Geometry check sheet. Reference: the model listing, model coordinates, mm. Round coordinates to 2 decimals unless told otherwise and drop trailing zeros. Write each loop counter-clockwise with the first axis right and the second up, starting at its lowest first coordinate (ties: lowest second). Pieces come first, ordered by that corner, then holes.
Item 1: Depth check by flat-ended pin: P1, Ø0.9, axis at y = -156, z = 1.5, coming from the +X side. Enter the tip coordinate at first touch or a pass-through.
Item 2: Scan lines: probe 1 along Y at (x, z) = (32.5, 2); probe 2 along Y at (x, z) = (8, 1.5); probe 3 along X at (y, z) = (-145, 2.05). Record each from-to range of solid material in increasing order.
Item 3: Cross-section at A-A (x = 46). Enter the section's corners in (y, z).
Item 4: Cross-section at B-B (y = -121.5). Enter the section's corners in (x, z).
Item 5: Cross-section at C-C (z = 1). State how many separate pieces and enclosed holes the cut face has, then the cut area to 3 significant figures.
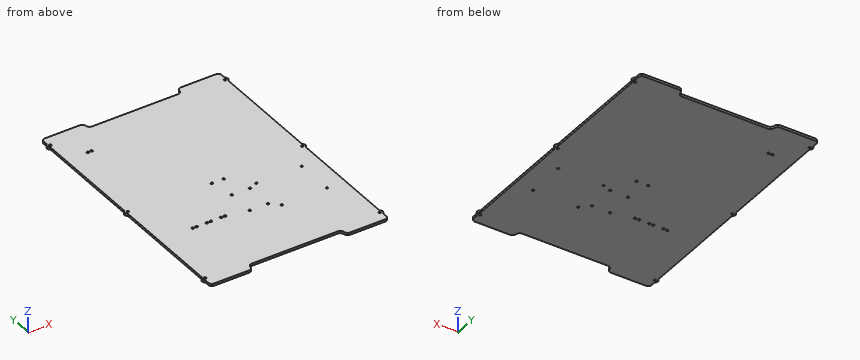
Autodesk Inventor part; units mm, degrees
ref_plane "YZ Plane" through (0, 0, 0) normal (1, 0, 0) x (0, 1, 0)
ref_plane "XZ Plane" through (0, 0, 0) normal (0, 1, 0) x (-1, 0, 0)
ref_plane "XY Plane" through (0, 0, 0) normal (0, 0, 1) x (1, 0, 0)
sketch "Sketch1" plane through (0, 0, 0) normal (0, 0, 1) x (1, 0, 0)
  line L0 (-114, -164) -> (114, -164)
  line L1 (114, 164) -> (-114, 164)
  line L2 (-114, -164) -> (114, 164) construction
  line L3 (114, -164) -> (-114, 164) construction
  line L4 (-112, -150) -> (112, -150)
  line L5 (112, -150) -> (112, 150)
  line L6 (112, 150) -> (-112, 150)
  line L7 (-112, 150) -> (-112, -150)
  line L8 (-112, -150) -> (112, 150) construction
  line L9 (112, -150) -> (-112, 150) construction
  circle A0 centre (112, 150) radius 1.5
  arc A1 (114, 146.5359) -> (114, 153.4641) centre (112, 150) ccw
  line L10 (114, 153.4641) -> (114, 164)
  line L11 (0, -56.7016) -> (0, 56.7016)
  line L12 (-37.0034, 0) -> (37.0034, 0)
  circle A2 centre (-112, 150) radius 1.5
  arc A3 (-114, 153.4641) -> (-114, 146.5359) centre (-112, 150) ccw
  circle A4 centre (112, -150) radius 1.5
  arc A5 (114, -153.4641) -> (114, -146.5359) centre (112, -150) ccw
  arc A6 (-114, -146.5359) -> (-114, -153.4641) centre (-112, -150) ccw
  circle A7 centre (-112, -150) radius 1.5
  line L13 (-114, 164) -> (-114, 153.4641)
  line L14 (114, -164) -> (114, -153.4641)
  line L15 (-114, -153.4641) -> (-114, -164)
  circle A8 centre (112, 0) radius 1.5
  arc A9 (114, -3.4641) -> (114, 3.4641) centre (112, 0) ccw
  line L16 (114, -146.5359) -> (114, -3.4641)
  line L17 (114, 3.4641) -> (114, 146.5359)
  circle A10 centre (-112, 0) radius 1.5
  arc A11 (-114, 3.4641) -> (-114, -3.4641) centre (-112, 0) ccw
  line L18 (-114, 146.5359) -> (-114, 3.4641)
  line L19 (-114, -3.4641) -> (-114, -146.5359)
  line L20 (-60, 164) -> (60, 164)
  line L21 (60, 164) -> (-60, 164)
  line L22 (-60, 164) -> (-60, 155)
  line L23 (-60, 155) -> (60, 155)
  line L24 (60, 155) -> (60, 164)
  line L25 (-60, -164) -> (-60, -155)
  line L26 (-60, -155) -> (60, -155)
  line L27 (60, -155) -> (60, -164)
  point P0 (0, 0)
  point P1 (0, 164)
  dimension "d0" = 228
  dimension "d1" = 328
  dimension "d2" = 224
  dimension "d3" = 300
  dimension "d4" = 3
  dimension "d10" = 3
  dimension "d11" = 8
  dimension "d12" = 120
  dimension "d13" = 120
  dimension "d14" = 9
extrude "Extrusion1" add sketch "Sketch1" along normal blind 3 contours L15 A6 L19 A11 L18 A3 L13 L1 L22 L23 L24 L10 A1 L17 A9 L16 A5 L14 L0 L27 L26 L25 | A7 L7 A10 A2 L6 A0 L5 A8 A4 L4
fillet "Fillet1" radius 4.1 4 edges at (114, 164, 1.5) (114, -164, 1.5) (-114, 164, 1.5) (-114, -164, 1.5)
fillet "Fillet2" radius 5 8 edges at (-60, 164, 1.5) (60, 164, 1.5) (60, 155, 1.5) (-60, 155, 1.5) (-60, -164, 1.5) (-60, -155, 1.5) (60, -155, 1.5) (60, -164, 1.5)
sketch "Sketch3" plane through (0, 0, 3) normal (0, 0, 1) x (1, 0, 0)
  circle A0 centre (-66.131, -64.28) radius 1.5
  circle A1 centre (-71.131, -64.28) radius 1.5
  circle A2 centre (-52.931, -64.28) radius 1.5
  circle A3 centre (-47.931, -64.28) radius 1.5
  circle A4 centre (-34.731, -64.28) radius 1.5
  circle A5 centre (-29.731, -64.28) radius 1.5
  circle A6 centre (-1.75, -35.23) radius 1.45
  circle A7 centre (21.55, -35.23) radius 1.45
  circle A8 centre (-1.75, -70.23) radius 1.45
  circle A9 centre (21.55, -70.23) radius 1.45
  circle A10 centre (32.5, -80.28) radius 1.35
  circle A11 centre (32.5, -31.28) radius 1.35
  circle A12 centre (90.5, -80.28) radius 1.35
  circle A13 centre (90.5, -31.28) radius 1.35
  circle A14 centre (-86.131, 116.72) radius 1.5
  circle A15 centre (-81.131, 116.72) radius 1.5
  circle A16 centre (-7.4766, -5.121) radius 1.5084
  circle A17 centre (7.5843, -5.1439) radius 1.4324
  point P0 (0, 0)
extrude "Extrusion3" cut sketch "Sketch3" against normal blind 3
properties part number "Control layer"
Resolved:
1. P1: stops at x = 114
2. probe 1: y = -155 to -81.63, -78.93 to -32.63, -29.93 to 155
2. probe 2: y = -155 to -6.51, -3.77 to 155
2. probe 3: x = -114 to 114
3. outline: (-155, 0) - (155, 0) - (155, 3) - (-155, 3) - close
4. outline: (-114, 0) - (114, 0) - (114, 3) - (-114, 3) - close
5. separate pieces: 1
5. enclosed holes: 24
5. area: 72,500 mm2
